Geometry check sheet. Reference: the model listing, model coordinates, mm. Face numbers are marked on the shaded views. Give positions to 0.01 mm unless a question says otherwise; leave off trailing zeros. Write each loop counter-clockwise with the first axis right and the second up, starting at its lowest first coordinate (ties: lowest second). Pieces come first, ordered by that corner, then holes. Notation, with made-up numbers: (-17.5, -25) -> (-3.5, -25) arc R24 ccw to (-3.5, 9) -> close; hole circle Ø6 at (52, 44). An arc over 180 degrees is marked (long way). Use a Markdown table: item, result. Add a question column.
from build123d import *

# Parameters (mm, degrees)
F0_W     = 186
F0_H     = 91
F1_DEPTH = 3
F2_W     = 182
F2_H     = 87
F2_W_2   = 178
F2_H_2   = 83
F3_DEPTH = 3
F4_W     = 8
F4_H     = 8
F5_DEPTH = 76
F6_W     = 4
F6_H     = 67
F6_W_2   = 162
F6_H_2   = 4
F7_DEPTH = 15


with BuildPart() as f1:
    # F0 (on Top) → F1 (new body)
    with BuildSketch(Plane.XY):
        Rectangle(F0_W, F0_H)
    extrude(amount=F1_DEPTH)

    # F2 (on face) → F3 (join)
    with BuildSketch(Plane(origin=(0, 0, 0), x_dir=(1, 0, 0), z_dir=(0, 0, -1))):
        Rectangle(F2_W, F2_H)
        Rectangle(F2_W_2, F2_H_2, mode=Mode.SUBTRACT)
    extrude(amount=F3_DEPTH)

    # F4 (on face) → F5 (join)
    with BuildSketch(Plane(origin=(0, 0, 0), x_dir=(1, 0, 0), z_dir=(0, 0, -1))):
        with Locations((-85, 37.5)):
            Rectangle(F4_W, F4_H)
        with Locations((-85, -37.5)):
            Rectangle(F4_W, F4_H)
        with Locations((85, 37.5)):
            Rectangle(F4_W, F4_H)
        with Locations((85, -37.5)):
            Rectangle(F4_W, F4_H)
    extrude(amount=F5_DEPTH)

    # F6 (on face) → F7 (join)
    with BuildSketch(Plane(origin=(0, 0, 0), x_dir=(1, 0, 0), z_dir=(0, 0, -1))):
        with Locations((83, 0)):
            Rectangle(F6_W, F6_H)
        with Locations((0, -35.5)):
            Rectangle(F6_W_2, F6_H_2)
        with Locations((-83, 0)):
            Rectangle(F6_W, F6_H)
        with Locations((0, 35.5)):
            Rectangle(F6_W_2, F6_H_2)
    extrude(amount=F7_DEPTH)


solid = f1.part
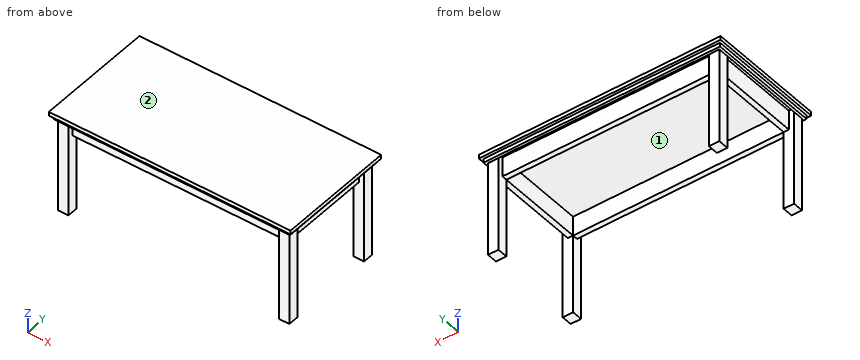
1) Gauge pin test, flat ends, axial feed: P1, Ø2.5, axis at y = 36.5, z = -36.5, coming from the +X side; P2, Ø7.5, axis at x = -4, z = -9.5, coming from the +Y side; P3, Ø1.5, axis at y = -6, z = -11, coming from the -X side. Record the tip position at first contact, or that the pin passes through.
2) Draft check along X on the marked faces 1 and 2. Enter one of: +X half, -X half, draft (parallel to the pull), parting line (faces both ways), or undercut.
3) Material ranges on probe 1 along Y at (x, z) = (-58, -9); probe 2 along X at (y, z) = (37, -54); probe 3 along Z at (x, y) = (84, -29.5), recorded low to high. Write a range as [from, to].
4) Sectioned sample at C-C, the plane y = 7. Enter the section's corners in (x, z).
5) Sectioned sample at A-A, the plane z = -31. Enter the section's corners in (x, y).
6) Sectioned sample at B-B, the plane x = 14. Enter the section's corners in (y, z).
Check values:
| question | item | result |
|---|---|---|
| 1 | P1 | x = 89 |
| 1 | P2 | y = 37.5 |
| 1 | P3 | x = -85 |
| 2 | face 1 | undercut |
| 2 | face 2 | draft |
| 3 | probe 1 | [-37.5, -33.5], [33.5, 37.5] |
| 3 | probe 2 | [-89, -81], [81, 89] |
| 3 | probe 3 | [-15, 3] |
| 4 | outline | (-93, 0) -> (-91, 0) -> (-91, -3) -> (-89, -3) -> (-89, 0) -> (-85, 0) -> (-85, -15) -> (-81, -15) -> (-81, 0) -> (81, 0) -> (81, -15) -> (85, -15) -> (85, 0) -> (89, 0) -> (89, -3) -> (91, -3) -> (91, 0) -> (93, 0) -> (93, 3) -> (-93, 3) -> close |
| 5 | outline | (-89, -41.5) -> (-81, -41.5) -> (-81, -33.5) -> (-89, -33.5) -> close; (-89, 33.5) -> (-81, 33.5) -> (-81, 41.5) -> (-89, 41.5) -> close; (81, -41.5) -> (89, -41.5) -> (89, -33.5) -> (81, -33.5) -> close; (81, 33.5) -> (89, 33.5) -> (89, 41.5) -> (81, 41.5) -> close |
| 6 | outline | (-45.5, 0) -> (-43.5, 0) -> (-43.5, -3) -> (-41.5, -3) -> (-41.5, 0) -> (-37.5, 0) -> (-37.5, -15) -> (-33.5, -15) -> (-33.5, 0) -> (33.5, 0) -> (33.5, -15) -> (37.5, -15) -> (37.5, 0) -> (41.5, 0) -> (41.5, -3) -> (43.5, -3) -> (43.5, 0) -> (45.5, 0) -> (45.5, 3) -> (-45.5, 3) -> close |
